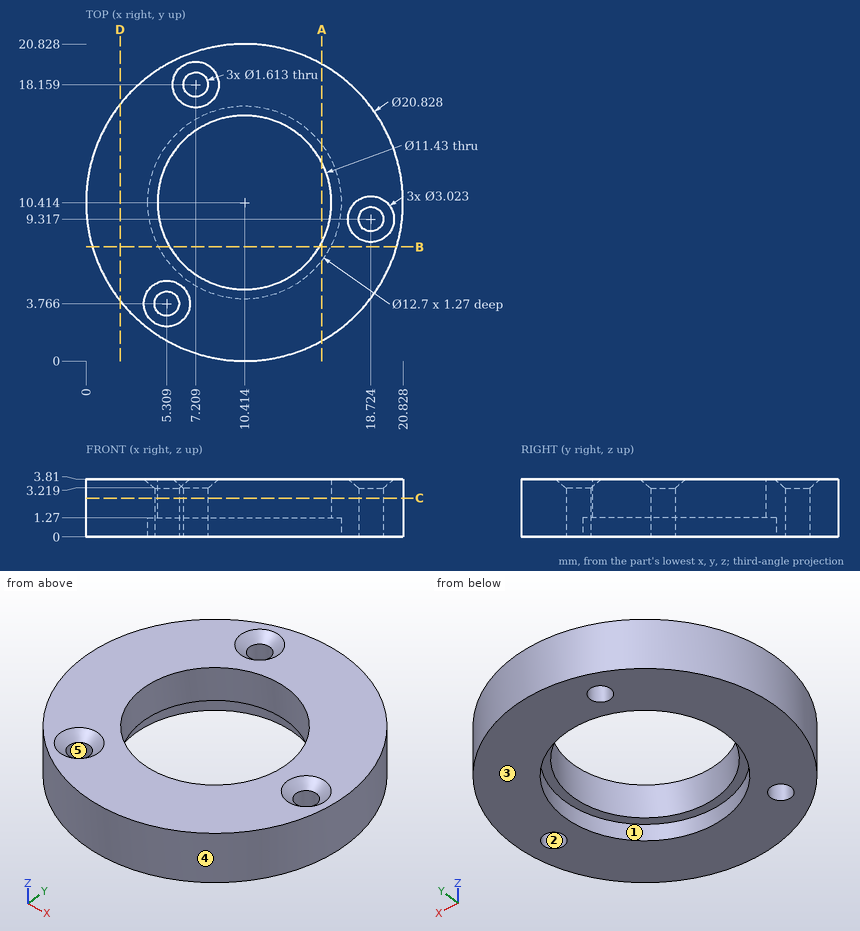
Here's the drawing with two shaded views (mm, measured from the low corner). I have some questions. A direction names the side the tool comes from. Coordinates: 2 decimals unless noted, no trailing zeros. Write each loop counter-clockwise with the first axis right and the second up, starting at its lowest first coordinate (ties: lowest second). Pieces come first, ordered by that corner, then holes. Notation, with made-up numbers: M -6,52.25 L 50,52.25 A17 cw 50,64.25 Z; hole C 18.5,-6.75 d4. An arc over 180 degrees is marked long. Use one line per item in the form item = value.
Q1. We'd pull the mould along X, two halves only. Please class the marked faces 3, 4 and 5: +X half, -X half, draft (parallel to the pull), parting line (faces both ways), or undercut.
Model answer:
face_3 = draft
face_4 = parting line
face_5 = undercut
Q2. I need wall thicknesses on line 1 along Y through (x, z) = (10.5, 2.2); line 2 along Y through (x, z) = (5.25, 1.3) (1 decimal); line 3 along Y through (x, z) = (7.25, 1.3) (1 decimal). Which ranges of each line are inside material? Lowest first, please. Write a range as from..to.
Model answer:
line_1 = 0..4.7, 16.13..20.83
line_2 = 1.4..3, 4.6..8, 12.9..19.5
line_3 = 0.5..5.7, 15.2..17.4, 19..20.3
Q3. If we section it at D-D (x = 2.25): Write out the boundary of the cut face in (y, z).
Model answer:
outline = M 3.95,0 L 16.88,0 L 16.88,3.81 L 3.95,3.81 Z
Q4. For the marked faces 1 and 2, which set-ups out of +Z, -Z, +X, -X, +Y, -Y let a thin tool reach every point of the face, with its end or its side?
Model answer:
face_1 = -Z
face_2 = +Z, -Z
Q5. If we section it at C-C (z = 2.55): Write out the boundary of the cut face in (x, y) (1 decimal), then the cut area to 3 significant figures.
Model answer:
outline = C 10.4,10.4 d20.8; hole C 5.3,3.8 d1.6; hole C 10.4,10.4 d11.4; hole C 7.2,18.2 d1.6; hole C 18.7,9.3 d1.6
area = 232 mm^2
Q6. If we section it at B-B (y = 7.5): Write out the boundary of the cut face in (x, z).
Model answer:
outline = M 0.42,0 L 4.77,0 L 4.77,1.27 L 5.5,1.27 L 5.5,3.81 L 0.42,3.81 Z; M 15.33,1.27 L 16.06,1.27 L 16.06,0 L 20.41,0 L 20.41,3.81 L 15.33,3.81 Z
Q7. If we section it at A-A (x = 15.5): Write out the boundary of the cut face in (y, z).
Model answer:
outline = M 1.33,0 L 6.61,0 L 6.61,1.27 L 7.81,1.27 L 7.81,3.81 L 1.33,3.81 Z; M 13.02,1.27 L 14.22,1.27 L 14.22,0 L 19.5,0 L 19.5,3.81 L 13.02,3.81 Z
Q8. For P1, Ø1, axis at x = 7.21, y = 18.16, coming from the +Z side, with a flat end and sliding along its axis, tell me the tip position at first contact or that it passes through.
Model answer:
P1 = through
